```python
from build123d import *

# Parameters (mm, degrees)
F1_DEPTH = 20
F2_R     = 1.5
F3_DEPTH = 5
F4_W     = 10
F4_H     = 4.2
F5_DEPTH = 5
F6_R     = 2.09999
F7_R     = 4.999


# Not quite as in the source:
# - a fillet or chamfer is up to 0.001 mm smaller than in the source, because OpenCascade refuses the exact size


with BuildPart() as f1:
    # F0 (on Right) → F1 (new body)
    with BuildSketch(Plane.YZ):
        with BuildLine():
            Line((76.2121204979, -15), (56.2121204979, -15))
            Line((56.2121204979, -15), (51.5942049014, -15))
            add(Edge.make_bspline(
                [(51.5942049014, -15), (51.5942049014, -16.6666666667), (51.5942043035, -18.3333333333), (51.5942049014, -20)],
                knots=[0, 0, 0, 0, 5, 5, 5, 5], degree=3))
            Line((51.5942049014, -20), (76.2121204979, -20))
            Line((76.2121204979, -20), (76.2121204979, -15))
        make_face()
        with BuildLine():
            Line((56.2121204979, -15), (56.2121204979, 0))
            Line((56.2121204979, 0), (47.2121204979, 0))
            add(Edge.make_bspline(
                [(47.2121204979, 0), (48.878788136, -3.0912153851), (50.9981620768, -11.3440190259), (51.5942049014, -15)],
                knots=[0, 0, 0, 0, 15.6269851129, 15.6269851129, 15.6269851129, 15.6269851129], degree=3))
            Line((51.5942049014, -15), (56.2121204979, -15))
        make_face()
        Polygon((56.2121204979, 0), (56.2121204979, 5), (-8.7878795021, 5), (-8.7878795021, 0), (47.2121204979, 0), align=None)
    extrude(amount=F1_DEPTH)

    # F2 (on face) → F3 (cut)
    with BuildSketch(Plane(origin=(0, 0, 0), x_dir=(1, 0, 0), z_dir=(0, 0, -1))):
        with Locations((10, -42.2121204979)):
            Circle(F2_R)
        with Locations((10, 3.7878795021)):
            Circle(F2_R)
    extrude(amount=-F3_DEPTH, mode=Mode.SUBTRACT)

    # F4 (on face) → F5 (cut)
    with BuildSketch(Plane.XY.offset(-15)):
        with Locations((10, 66.2121204979)):
            Rectangle(F4_W, F4_H)
    extrude(amount=-F5_DEPTH, mode=Mode.SUBTRACT)

    # F6 (radius 2.1 in the source; OpenCascade refuses exactly that, so slightly less here)
    f6_edges = [f1.edges().sort_by_distance(p)[0] for p in [
        (5, 68.31212, -17.5),
        (15, 68.31212, -17.5),
        (15, 64.11212, -17.5),
        (5, 64.11212, -17.5),
    ]]
    fillet(f6_edges, radius=F6_R)

    # F7 (radius 5 in the source; OpenCascade refuses exactly that, so slightly less here)
    f7_edges = [f1.edges().sort_by_distance(p)[0] for p in [
        (10, 56.21212, 5),
        (10, 76.21212, -20),
        (10, 51.594205, -20),
    ]]
    fillet(f7_edges, radius=F7_R)


solid = f1.part
```
Check sheet for the modelled part. Datum: model origin and axes. Units: mm. A direction names the side the tool comes from. Round coordinates to 2 decimals unless told otherwise and drop trailing zeros. Write each loop counter-clockwise with the first axis right and the second up, starting at its lowest first coordinate (ties: lowest second). Pieces come first, ordered by that corner, then holes. Notation, with made-up numbers: M -15,44 L 14,44 A18 ccw 14,63 Z; hole C 87,60.25 d7. An arc over 180 degrees is marked long. Write item = value, one per line. Start each with the question number.
1. Scan lines: line 1 (Y direction, x = 10, z = 1.2); line 2 (Y direction, x = 10, z = 1.6); line 3 (Z direction, x = 2.5, y = 65). Record each from-to range of solid material in increasing order. Write a range as [from, to].
2. Tool access check on faces 1 (the cylindrical face through (14, 68, -18)), 2 (the flat face through (10, 19, 0)), 3 (the flat face through (10, 56.212, -8)), 4 (the cylindrical face through (10.14, 74.787, -18.497)), 5 (the flat face through (0, 37, 1)). Record the directions out of +Z, -Z, +X, -X, +Y, -Y that give a thin tool (end or side, any length) a straight path to the whole face; none if there is none.
3. Section check A-A, the plane y = 58.5. Record the cut outline in (x, z).
4. Section check B-B, the plane x = 10. State how many separate pieces and enclosed holes the cut face has, then the cut area to 3 significant figures.
5. Gauge pin test, flat ends, axial feed: pin 1 (5 mm diameter, centred on x = 7, y = 25, fed in from -Z); pin 2 (4.5 mm diameter, centred on x = 10.5, z = -7, fed in from +Y); pin 3 (1.5 mm diameter, centred on x = 9, z = -18.5, fed in from -Y); pin 4 (12 mm diameter, centred on x = 11.5, z = -11, fed in from +Y). Record the tip position at first contact, or that the pin passes through.
6. Release check for a two-part mould opening along Y. For faces 6 (the flat face through (10, 68.312, -17)), 7 (the cylindrical face through (6, 68, -18)), 8 (the flat face through (10, -8.788, 3)), 9 (the flat face through (10, 22, 5)) record: pulls with the +Y half, pulls with the -Y half, needs draft (parallel to the pull), parting line crosses it, or undercut.
Results found:
q1.line_1 = [-8.79, -5.29], [-2.29, 40.71], [43.71, 56.07]
q1.line_2 = [-8.79, -5.29], [-2.29, 40.71], [43.71, 55.95]
q1.line_3 = [-20, -15]
q2.face_1 = +Z, -Z
q2.face_2 = -Z, +X, -X, -Y
q2.face_3 = +Z, +X, -X, +Y
q2.face_4 = -Z, +X, -X, +Y
q2.face_5 = +Z, -Z, -X, +Y, -Y
q3.outline = M 0,-20 L 20,-20 L 20,-15 L 0,-15 Z
q4.separate_pieces = 4
q4.enclosed_holes = 0
q4.area = 478 mm^2
q5.pin_1 = 0
q5.pin_2 = 56.21
q5.pin_3 = 52.42
q5.pin_4 = 76.21
q6.face_6 = undercut
q6.face_7 = undercut
q6.face_8 = pulls with the -Y half
q6.face_9 = needs draft
